from build123d import *

# Parameters (mm, degrees)
EXTRUDE_1_DEPTH        = 510
SKETCH_2_W             = 15
SKETCH_2_H             = 15
EXTRUDE_2_DEPTH        = 15
PATTERN_LINEAR_1_COUNT = 2
PATTERN_LINEAR_1_PITCH = 495


with BuildPart() as part:
    # Эскиз1 → Бобышка-Вытянуть1 (new body)
    with BuildSketch(Plane.XY):
        Polygon((0, 0), (15, 0), (15, 15), (30, 15), (30, 170), (0, 170), align=None)
    extrude(amount=EXTRUDE_1_DEPTH)

    # Эскиз2 → Бобышка-Вытянуть2 (add)
    with BuildSketch(Plane(origin=(0, 0, 0), x_dir=(-1, 0, 0), z_dir=(0, 0, -1))):
        with Locations((-22.5, 7.5)):
            Rectangle(SKETCH_2_W, SKETCH_2_H)
    extrude_2 = extrude(amount=-EXTRUDE_2_DEPTH)

    # Линейный массив1: Бобышка-Вытянуть2 ×2
    with Locations(*[(0, 0, i * PATTERN_LINEAR_1_PITCH) for i in range(1, PATTERN_LINEAR_1_COUNT)]):
        add(extrude_2)


solid = part.part
The model under review builds one solid part; all positions refer to its coordinate system, in mm. A direction names the side the tool comes from. Coordinates: 2 decimals unless noted, no trailing zeros. Loops run counter-clockwise (first coordinate to the right, second up) from the corner with the lowest first, then second, coordinate; pieces in that order, holes last. Notation, with made-up numbers: M 7,48.5 L 14,48.5 A23 ccw 14,62.5 Z; hole C 37,-39 d7. An arc over 180 degrees is marked long. Put each result on its own line as item: value. Start each with the question number.
Q1. The part is to be moulded in two halves that separate along Z. For faces 3 (the flat face through (15, 86, 510)), 4 (the flat face through (30, 84, 251)), 5 (the flat face through (15, 86, 0)), 6 (the flat face through (15, 7, 252)), say which applies: +Z half, -Z half, draft (parallel to the pull), parting line (faces both ways), or undercut.
Q2. Clearance check with a flat-ended pin moving along its axis: pin 1 (8 mm diameter, centred on x = 20, z = 399.5, fed in from -Y). State where the tip first meets the part, or that it passes through.
Q3. For faces 1 (the flat face through (22, 15, 252)), 2 (the flat face through (15, 170, 251)), list the 3-axis set-ups (+Z, -Z, +X, -X, +Y, -Y) from which the entire face can be reached by the end or side of a thin tool; tool diameter is ignored.
Q4. Add section A-A (z = 100). Write out the cut boundary in (x, y).
Q5. Wall thickness on line 1 (Y direction, x = 22.5, z = 52); line 2 (X direction, y = 7.5, z = 283): over which ranges is each line inside the solid? List them lowest first.
Answers:
1. face 3: +Z half
1. face 4: draft
1. face 5: -Z half
1. face 6: undercut
2. pin 1: stops at y = 15
3. face 1: +X, -Y
3. face 2: +Z, -Z, +X, -X, +Y
4. outline: M 0,0 L 15,0 L 15,15 L 30,15 L 30,170 L 0,170 Z
5. line 1: y = 15 to 170
5. line 2: x = 0 to 15
